Autodesk Inventor part; units mm, degrees
ref_plane "aluschild_XY" through (0, 0, 0) normal (0, 0, 1) x (1, 0, 0)
ref_plane "aluschild_YZ" through (0, 0, 0) normal (1, 0, 0) x (0, 1, 0)
ref_plane "aluschild_ZX" through (0, 0, 0) normal (0, 1, 0) x (0, 0, 1)
sketch "Sketch_1" plane through (0, 0, 0) normal (0, 0, 1) x (1, 0, 0)
  arc A0 (-12, 0) -> (-7.5, -4.5) centre (-7.5, 0) ccw
  line L0 (-7.5, -4.5) -> (7.5, -4.5)
  arc A1 (7.5, -4.5) -> (12, 0) centre (7.5, 0) ccw
  arc A2 (12, 0) -> (7.5, 4.5) centre (7.5, 0) ccw
  line L1 (7.5, 4.5) -> (-7.5, 4.5)
  arc A3 (-7.5, 4.5) -> (-12, 0) centre (-7.5, 0) ccw
extrude "Extrusion1" add sketch "Sketch_1" along normal blind 0.3
sketch "Sketch_13" plane through (0, 0, 0.3) normal (0, 0, 1) x (1, 0, 0)
  line L0 (-5.2261, 1.0265) -> (-5.2261, -1.027)
  line L1 (-5.2261, -1.027) -> (-4.5423, -1.027)
  line L2 (-4.5423, -1.027) -> (-4.5423, -0.2502)
  line L3 (-4.5423, -0.2502) -> (-3.7899, -0.2502)
  line L4 (-3.7899, -0.2502) -> (-3.7899, -1.027)
  line L5 (-3.7899, -1.027) -> (-3.106, -1.027)
  line L6 (-3.106, -1.027) -> (-3.106, 1.0265)
  line L7 (-3.106, 1.0265) -> (-3.7899, 1.0265)
  line L8 (-3.7899, 1.0265) -> (-3.7899, 0.2798)
  line L9 (-3.7899, 0.2798) -> (-4.5423, 0.2798)
  line L10 (-4.5423, 0.2798) -> (-4.5423, 1.0265)
  line L11 (-4.5423, 1.0265) -> (-5.2261, 1.0265)
extrude "Extrusion2" cut sketch "Sketch_13" against normal blind 0.05
sketch "Sketch_15" plane through (0, 0, 0.3) normal (0, 0, 1) x (1, 0, 0)
  line L0 (-0.689, 1.0265) -> (-0.689, -1.027)
  line L1 (-0.689, -1.027) -> (-0.0337, -1.027)
  line L2 (-0.0337, -1.027) -> (-0.0337, 0.0269)
  line L3 (-0.0337, 0.0269) -> (0.9535, -1.027)
  line L4 (0.9535, -1.027) -> (1.537, -1.027)
  line L5 (1.537, -1.027) -> (1.537, 1.0265)
  line L6 (1.537, 1.0265) -> (0.8819, 1.0265)
  line L7 (0.8819, 1.0265) -> (0.8819, -0.0273)
  line L8 (0.8819, -0.0273) -> (-0.1051, 1.0265)
  line L9 (-0.1051, 1.0265) -> (-0.689, 1.0265)
extrude "Extrusion3" cut sketch "Sketch_15" against normal blind 0.05
sketch "Sketch_16" plane through (0, 0, 0.3) normal (0, 0, 1) x (1, 0, 0)
  line L0 (1.7129, 1.0265) -> (1.7129, -1.027)
  line L1 (1.7129, -1.027) -> (2.3967, -1.027)
  line L2 (2.3967, -1.027) -> (2.3967, -0.0588)
  line L3 (2.3967, -0.0588) -> (3.1093, -1.027)
  line L4 (3.1093, -1.027) -> (3.9246, -1.027)
  line L5 (3.9246, -1.027) -> (3.1004, 0.0719)
  line L6 (3.1004, 0.0719) -> (3.8959, 1.0265)
  line L7 (3.8959, 1.0265) -> (3.1777, 1.0265)
  line L8 (3.1777, 1.0265) -> (2.3967, 0.0961)
  line L9 (2.3967, 0.0961) -> (2.3967, 1.0265)
  line L10 (2.3967, 1.0265) -> (1.7129, 1.0265)
extrude "Extrusion4" cut sketch "Sketch_16" against normal blind 0.05
sketch "Sketch_5" plane through (0, 0, 0.3) normal (0, 0, 1) x (1, 0, 0)
  arc A0 (-8.6625, 0.2585) -> (-8.1925, -0.2115) centre (-8.1925, 0.2585) ccw
  line L0 (-8.1925, -0.2115) -> (-7.9457, -0.2115)
  arc A1 (-7.9457, -0.611) -> (-7.9457, -0.2115) centre (-7.9457, -0.4113) ccw
  line L1 (-7.9457, -0.611) -> (-8.6625, -0.611)
  line L2 (-8.6625, -0.611) -> (-8.6625, -1.0575)
  line L3 (-8.6625, -1.0575) -> (-7.9105, -1.0575)
  arc A2 (-7.9105, -1.0575) -> (-7.2525, -0.3995) centre (-7.9105, -0.3995) ccw
  line L4 (-7.2525, -0.3995) -> (-7.2525, -0.2585)
  arc A3 (-7.2525, -0.2585) -> (-7.7225, 0.2115) centre (-7.7225, -0.2585) ccw
  line L5 (-7.7225, 0.2115) -> (-7.9457, 0.2115)
  arc A4 (-7.9457, 0.611) -> (-7.9457, 0.2115) centre (-7.9395, 0.4113) ccw
  line L6 (-7.9457, 0.611) -> (-7.2525, 0.611)
  line L7 (-7.2525, 0.611) -> (-7.2525, 1.0575)
  line L8 (-7.2525, 1.0575) -> (-8.0045, 1.0575)
  arc A5 (-8.0045, 1.0575) -> (-8.6625, 0.3995) centre (-8.0045, 0.3995) ccw
  line L9 (-8.6625, 0.3995) -> (-8.6625, 0.2585)
extrude "Extrusion5" cut sketch "Sketch_5" against normal blind 0.05
sketch "Sketch_6" plane through (0, 0, 0.3) normal (0, 0, 1) x (1, 0, 0)
  arc A0 (-6.04, 1.0693) -> (-6.04, -1.0693) centre (-6.04, 0) ccw
  line L0 (-6.04, -1.0693) -> (-5.429, -1.0693)
  line L1 (-5.429, -1.0693) -> (-5.429, -0.3995)
  line L2 (-5.429, -0.3995) -> (-6.04, -0.3995)
  arc A1 (-6.04, 0.3995) -> (-6.04, -0.3995) centre (-6.04, 0) ccw
  line L3 (-6.04, 0.3995) -> (-5.429, 0.3995)
  line L4 (-5.429, 0.3995) -> (-5.429, 1.0693)
  line L5 (-5.429, 1.0693) -> (-6.04, 1.0693)
extrude "Extrusion6" cut sketch "Sketch_6" against normal blind 0.05
sketch "Sketch_7" plane through (0, 0, 0.3) normal (0, 0, 1) x (1, 0, 0)
  line L0 (-2.948, 1.034) -> (-2.948, 0)
  arc A0 (-2.948, 0) -> (-0.833, 0) centre (-1.8905, 0) ccw
  line L1 (-0.833, 0) -> (-0.833, 1.034)
  line L2 (-0.833, 1.034) -> (-1.5145, 1.034)
  line L3 (-1.5145, 1.034) -> (-1.5145, 0)
  arc A1 (-2.2665, 0) -> (-1.5145, 0) centre (-1.8905, 0) ccw
  line L4 (-2.2665, 0) -> (-2.2665, 1.034)
  line L5 (-2.2665, 1.034) -> (-2.948, 1.034)
extrude "Extrusion7" cut sketch "Sketch_7" against normal blind 0.05
sketch "Sketch8" plane through (0, 0, 0.3) normal (0, 0, 1) x (1, 0, 0)
  point P0 (6.6, 0)
hole "Hole1" at (6.6, 0, 0.3) direction (0, 0, -1) diameter 1.344 depth 0.05
sketch "Sketch_3" plane through (0, 0, 0.3) normal (0, 0, 1) x (1, 0, 0)
  arc A0 (7.2909, 2.2698) -> (4.4594, -1.0234) centre (6.6, 0) ccw
  line L0 (4.4594, -1.0234) -> (5.7362, -0.352)
  arc A1 (7.3714, 0.5243) -> (5.7362, -0.352) centre (6.6, 0) ccw
  line L1 (7.3714, 0.5243) -> (8.9464, 1.3615)
  line L2 (8.9464, 1.3615) -> (8.9464, 3.1479)
  line L3 (8.9464, 3.1479) -> (7.2909, 2.2698)
extrude "Extrusion8" cut sketch "Sketch_3" against normal blind 0.05
sketch "Sketch_4" plane through (0, 0, 0.3) normal (0, 0, 1) x (1, 0, 0)
  line L0 (4.262, -1.3559) -> (4.262, -3.1423)
  line L1 (4.262, -3.1423) -> (5.9182, -2.2715)
  arc A0 (5.9182, -2.2715) -> (8.7347, 1.0332) centre (6.6, 0) ccw
  line L2 (8.7347, 1.0332) -> (7.4617, 0.3479)
  arc A1 (5.8342, -0.5264) -> (7.4617, 0.3479) centre (6.6, 0) ccw
  line L3 (5.8342, -0.5264) -> (4.262, -1.3559)
extrude "Extrusion9" cut sketch "Sketch_4" against normal blind 0.05
ref_plane "aluschild_XY" through (0, 0, 0) normal (0, 0, 1) x (1, 0, 0)
ref_plane "aluschild_YZ" through (0, 0, 0) normal (1, 0, 0) x (0, 1, 0)
ref_plane "aluschild_ZX" through (0, 0, 0) normal (0, 1, 0) x (0, 0, 1)
properties part number "SCHUNK-9905502 Typenschild 9x24x0.3"
The model under review builds one solid part; all positions refer to its coordinate system, in mm. A direction names the side the tool comes from. Give positions to 0.01 mm unless a question says otherwise; leave off trailing zeros. Write each loop counter-clockwise with the first axis right and the second up, starting at its lowest first coordinate (ties: lowest second). Pieces come first, ordered by that corner, then holes. Notation, with made-up numbers: (74, -1) -> (123, -1) arc R24 ccw to (123, 32) -> close; hole circle Ø7 at (-34.75, -36.75). An arc over 180 degrees is marked (long way). Answer in a Markdown table with one row per item.
1) Add section B-B on x = 10.75. State the section outline as (y, z) points, plus the area to 3 significant figures.
Worked answers:
| item | result |
|---|---|
| outline | (-3.11, 0) -> (3.11, 0) -> (3.11, 0.3) -> (-3.11, 0.3) -> close |
| area | 1.87 mm² |
2) For L1, parallel to Z at x = 7.5, y = 2; L2, parallel to X at y = -1.5, z = 0.2; L3, parallel to X at y = -0.5, z = 0.15, list the stretches that pass through material, from the lowest coordinate up. Write a range as [from, to].
Worked answers:
| item | result |
|---|---|
| L1 | [0, 0.25] |
| L2 | [-11.74, 11.74] |
| L3 | [-11.97, 11.97] |
3) Add section A-A on y = -1.75. State the section outline as (x, z) points.
Worked answers:
| item | result |
|---|---|
| outline | (-11.65, 0) -> (11.65, 0) -> (11.65, 0.3) -> (8.2, 0.3) -> (8.2, 0.25) -> (4.26, 0.25) -> (4.26, 0.3) -> (-11.65, 0.3) -> close |
4) Add section C-C on y = 3.5. State the section outline as (x, z) points, plus the area to 3 significant figures.
Worked answers:
| item | result |
|---|---|
| outline | (-10.33, 0) -> (10.33, 0) -> (10.33, 0.3) -> (-10.33, 0.3) -> close |
| area | 6.20 mm² |
5) Tool access review of faces 4 (the flat face through (-8, 0, 0.25)), 5 (the cylindrical face through (12, 0.1, 0.15)): name each direction out of +Z, -Z, +X, -X, +Y, -Y from which nothing blocks a thin tool from reaching the whole face with its end or side.
Worked answers:
| item | result |
|---|---|
| face 4 | +Z |
| face 5 | +Z, -Z, +X |
6) Mouldability with a two-part tool opening along Y and no side actions: class faces 1 (the flat face through (0, 2, 0.3)), 2 (the cylindrical face through (-12, -0.1, 0.15)), 3 (the flat face through (7, 0, 0.25)) as +Y half, -Y half, draft (parallel to the pull), parting line (faces both ways), or undercut.
Worked answers:
| item | result |
|---|---|
| face 1 | draft |
| face 2 | parting line |
| face 3 | undercut |
